Input: part model. Units: mm. Frame: model coordinates. Face numbers are marked on the shaded views. Give positions to 0.01 mm unless a question says otherwise; leave off trailing zeros. Loops run counter-clockwise (first coordinate to the right, second up) from the corner with the lowest first, then second, coordinate; pieces in that order, holes last. Notation, with made-up numbers: (68, -23) - (118, -23) arc R10 ccw to (118, -5) - close; hole circle Ø10 at (55.25, 39.25). An arc over 180 degrees is marked (long way). One line per item, written item: value.
from build123d import *

# Parameters (mm, degrees)
F0_R     = 11.25
F1_DEPTH = 21
F0_R_2   = 12.5
F2_DEPTH = 1
F3_R     = 6.5
F4_DEPTH = 19


with BuildPart() as f1:
    # F0 (on Top) → F1 (new body)
    with BuildSketch(Plane.XY):
        Circle(F0_R)
    extrude(amount=F1_DEPTH)

    # F0 (on Top) → F2 (join)
    with BuildSketch(Plane.XY):
        Circle(F0_R_2)
        Circle(F0_R, mode=Mode.SUBTRACT)
    extrude(amount=F2_DEPTH)

    # F3 (on face) → F4 (cut)
    with BuildSketch(Plane(origin=(0, 0, 0), x_dir=(1, 0, 0), z_dir=(0, 0, -1))):
        Circle(F3_R)
    extrude(amount=-F4_DEPTH, mode=Mode.SUBTRACT)


solid = f1.part
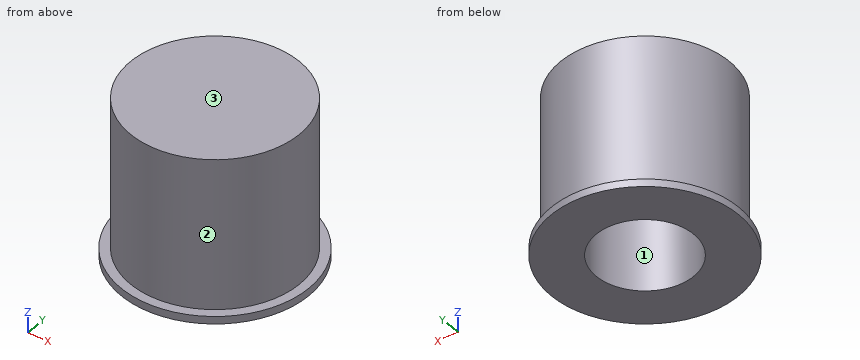
Item 1: Section A-A, the plane y = 0. Output: boundary loops of the cut face in (x, z), and give its area (3 significant figures).
Verdict:
outline: (-12.5, 0) - (-6.5, 0) - (-6.5, 19) - (6.5, 19) - (6.5, 0) - (12.5, 0) - (12.5, 1) - (11.25, 1) - (11.25, 21) - (-11.25, 21) - (-11.25, 1) - (-12.5, 1) - close
area: 228 mm^2
Item 2: Material intervals for L1, parallel to Y at x = 0, z = 5.25; L2, parallel to Z at x = -1.5, y = 1.75; L3, parallel to Z at x = 6.5, y = -9.75, sorted ascending.
Verdict:
L1: y = -11.25 to -6.5, 6.5 to 11.25
L2: z = 19 to 21
L3: z = 0 to 1
Item 3: Pin query (flat end, axial travel): P1, Ø12, axis at x = -0.5, z = 17.5, coming from the -Y side; P2, Ø8, axis at x = -9.5, z = 4, coming from the +Y side; P3, Ø10, axis at y = 8, z = 9.5, coming from the +X side. Return the tip coordinate at first contact, or that it passes through.
Verdict:
P1: stops at y = -11.25
P2: stops at y = 10.45
P3: stops at x = 10.84
Item 4: Draft query along Y for the marked faces 1, 2 and 3. Return one class per face: pulls with the +Y half, pulls with the -Y half, needs draft (parallel to the pull), parting line crosses it, or undercut.
Verdict:
face 1: undercut
face 2: parting line crosses it
face 3: needs draft
Item 5: Section D-D, the plane y = 9.5. Output: boundary loops of the cut face in (x, z), and give its area (3 significant figures).
Verdict:
outline: (-8.12, 0) - (8.12, 0) - (8.12, 1) - (6.03, 1) - (6.03, 21) - (-6.03, 21) - (-6.03, 1) - (-8.12, 1) - close
area: 257 mm^2
Item 6: Section B-B, the plane z = 12.25. Output: boundary loops of the cut face in (x, y), and give its area (3 significant figures).
Verdict:
outline: circle Ø22.5 at (0, 0); hole circle Ø13 at (0, 0)
area: 265 mm^2
